Geometry check sheet. Reference: the model listing, model coordinates, mm. A direction names the side the tool comes from. Coordinates: 2 decimals unless noted, no trailing zeros. Loops run counter-clockwise (first coordinate to the right, second up) from the corner with the lowest first, then second, coordinate; pieces in that order, holes last.
from build123d import *

# Parameters (mm, degrees)
F0_W     = 300
F0_H     = 100
F1_DEPTH = 50
F3_W     = 10
F3_H     = 10
F4_DEPTH = 300


with BuildPart() as f1:
    # F0 (on Top) → F1 (new body, symmetric)
    with BuildSketch(Plane.XY):
        Rectangle(F0_W, F0_H)
    extrude(amount=F1_DEPTH, both=True)

    # F3 (on face) → F4 (join)
    with BuildSketch(Plane(origin=(-150, 0, 0), x_dir=(0, -1, 0), z_dir=(-1, 0, 0))):
        with Locations((35, 55)):
            Rectangle(F3_W, F3_H)
        with Locations((-35, 55)):
            Rectangle(F3_W, F3_H)
    extrude(amount=-F4_DEPTH)


solid = f1.part
(1) Gauge pin test, flat ends, axial feed: pin 1 Ø5 at (x, z) = (-43, 54.5) entering from +Y; pin 2 Ø5 at (x, z) = (-16.5, 53.5) entering from -Y; pin 3 Ø8 at (x, y) = (44, 45.5) entering from +Z. Record the tip position at first contact, or that the pin passes through.
Findings:
pin 1: stops at y = 40
pin 2: stops at y = -40
pin 3: stops at z = 50
(2) Sectioned sample at A-A on x = 101. Record the cut outline in (y, z), and give its area (3 significant figures).
Findings:
outline: (-50, -50) - (50, -50) - (50, 50) - (40, 50) - (40, 60) - (30, 60) - (30, 50) - (-30, 50) - (-30, 60) - (-40, 60) - (-40, 50) - (-50, 50) - close
area: 10,200 mm2
(3) Draft check along Y on faces 4 (the flat face through (-2, 45, 50)), 5 (the flat face through (-2, 40, 55)), 6 (the flat face through (-2, 0, 50)), 7 (the flat face through (-2, 30, 55)). Enter one of: +Y half, -Y half, draft (parallel to the pull), parting line (faces both ways), or undercut.
Findings:
face 4: draft
face 5: +Y half
face 6: undercut
face 7: undercut
(4) Access from +Z, -Z, +X, -X, +Y, -Y to the whole of each face (thin tool, end or side, straight path). Record for faces 1 (the flat face through (-2, -45, 50)), 2 (the flat face through (-2, -30, 55)), 3 (the flat face through (-2, -50, 1)).
Findings:
face 1: +Z, +X, -X, -Y
face 2: +Z, +X, -X
face 3: +Z, -Z, +X, -X, -Y
(5) Scan lines: L1, parallel to Y at x = -41.5, z = 54; L2, parallel to Z at x = -86, y = 17.5. Record each from-to range of solid material in increasing order.
Findings:
L1: y = -40 to -30, 30 to 40
L2: z = -50 to 50
(6) Sectioned sample at B-B on y = 14. Record the cut outline in (x, z), and give its area (3 significant figures).
Findings:
outline: (-150, -50) - (150, -50) - (150, 50) - (-150, 50) - close
area: 30,000 mm2
